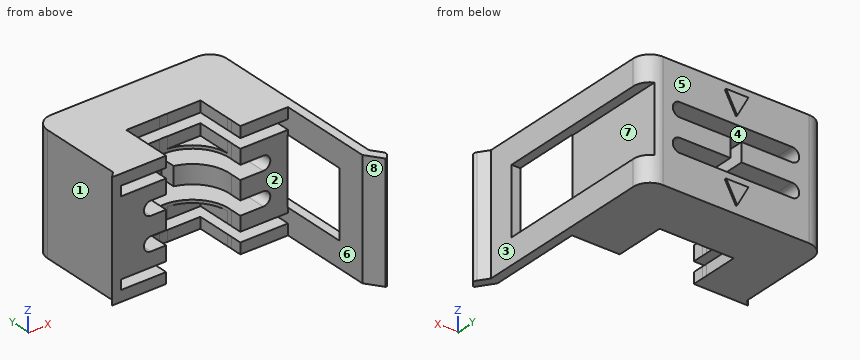
from build123d import *

# Parameters (mm, degrees)
SALIENTE_EXTRUIR1_DEPTH = 21.02
CORTAR_EXTRUIR1_DEPTH   = 48.423848102
SALIENTE_EXTRUIR2_DEPTH = 0.3
CORTAR_EXTRUIR2_DEPTH   = 1.7
CROQUIS6_W              = 13.32
CROQUIS6_H              = 9.1
CORTAR_EXTRUIR3_DEPTH   = 5.78
CROQUIS7_W              = 13.32
CROQUIS7_H              = 9.1
CORTAR_EXTRUIR4_DEPTH   = 5.78
CROQUIS8_W              = 21.89
CROQUIS8_H              = 1.74582909
CORTAR_EXTRUIR5_DEPTH   = 15.76


with BuildPart() as part:
    # Croquis2 → Saliente-Extruir1 (new body)
    with BuildSketch(Plane.XY):
        with BuildLine():
            Line((16.1, -25.6), (16.1, -9.1))
            Line((16.1, -9.1), (16.1, 6.87))
            ThreePointArc((16.1, 6.87), (15.221320344, 8.991320344), (13.1, 9.87))
            Line((13.1, 9.87), (-13.1, 9.87))
            ThreePointArc((-13.1, 9.87), (-15.221320344, 8.991320344), (-16.1, 6.87))
            Line((-16.1, 6.87), (-16.1, -8.084842917))
            Line((-16.1, -8.084842917), (-17.1, -9.1))
            Line((-17.1, -9.1), (-16.1, -9.1))
            Line((-16.1, -9.1), (-7.36, -9.1))
            Line((-7.36, -9.1), (-7.36, -7.1))
            ThreePointArc((-7.36, -7.1), (-0.7, 0.036800452), (5.96, -7.1))
            Line((5.96, -7.1), (5.96, -9.1))
            Line((5.96, -9.1), (14.53, -9.1))
            Line((14.53, -9.1), (14.53, -26.095019099))
            Line((14.53, -26.095019099), (16.46294155, -28.855545721))
            ThreePointArc((16.46294155, -28.855545721), (16.646307517, -28.898064095), (16.810355034, -28.805764032))
            Line((16.810355034, -28.805764032), (16.821593757, -28.791058008))
            Line((16.821593757, -28.791058008), (17.28495009, -28.184749839))
            ThreePointArc((17.28495009, -28.184749839), (17.43599966, -27.735907903), (17.281999232, -27.288069848))
            Line((17.281999232, -27.288069848), (16.1, -25.6))
        make_face()
    extrude(amount=SALIENTE_EXTRUIR1_DEPTH)

    # Croquis3 → Cortar-Extruir1 (cut, through all)
    with BuildSketch(Plane(origin=(0, 9.87, 0), x_dir=(1, 0, 0), z_dir=(0, 1, 0))):
        with BuildLine():
            Line((-10.1, -12.17), (-1, -12.17))
            Line((-1, -12.17), (-1, -8.83))
            Line((-1, -8.83), (-10.1, -8.83))
            ThreePointArc((-10.1, -8.83), (-11.35, -7.58), (-10.1, -6.33))
            Line((-10.1, -6.33), (10.1, -6.33))
            ThreePointArc((10.1, -6.33), (11.35, -7.58), (10.1, -8.83))
            Line((10.1, -8.83), (1, -8.83))
            Line((1, -8.83), (1, -12.17))
            Line((1, -12.17), (10.1, -12.17))
            ThreePointArc((10.1, -12.17), (11.35, -13.42), (10.1, -14.67))
            Line((10.1, -14.67), (-10.1, -14.67))
            ThreePointArc((-10.1, -14.67), (-11.35, -13.42), (-10.1, -12.17))
        make_face()
    extrude(amount=-CORTAR_EXTRUIR1_DEPTH, mode=Mode.SUBTRACT)

    # Croquis4 → Saliente-Extruir2 (add)
    with BuildSketch(Plane(origin=(0, 9.87, 0), x_dir=(-1, 0, 0), z_dir=(0, 1, 0))):
        Polygon((0, 16.02), (2, 19.67), (-2, 19.67), align=None)
        Polygon((2, 4.98), (-2, 4.98), (0, 1.33), align=None)
    extrude(amount=SALIENTE_EXTRUIR2_DEPTH)

    # Croquis5 → Cortar-Extruir2 (cut)
    with BuildSketch(Plane(origin=(16.1, 0, 0), x_dir=(0, 0, -1), z_dir=(1, 0, 0))):
        Polygon((-16.46, 6.87), (-16.46, -20.9), (-10.51, -20.9), (-4.56, -20.9), (-4.56, 6.87), align=None)
        Polygon((-16.46, 9.815378902), (-16.46, 6.87), (-4.56, 6.87), (-4.56, 10.17), align=None)
    extrude(amount=-CORTAR_EXTRUIR2_DEPTH, mode=Mode.SUBTRACT)

    # Croquis6 → Cortar-Extruir3 (cut)
    with BuildSketch(Plane(origin=(0, 0, 0), x_dir=(-1, 0, 0), z_dir=(0, 0, -1))):
        with Locations((0.7, -4.55)):
            Rectangle(CROQUIS6_W, CROQUIS6_H)
    extrude(amount=-CORTAR_EXTRUIR3_DEPTH, mode=Mode.SUBTRACT)

    # Croquis7 → Cortar-Extruir4 (cut)
    with BuildSketch(Plane.XY.offset(21.02)):
        with Locations((-0.7, -4.55)):
            Rectangle(CROQUIS7_W, CROQUIS7_H)
    extrude(amount=-CORTAR_EXTRUIR4_DEPTH, mode=Mode.SUBTRACT)

    # Croquis8 → Cortar-Extruir5 (cut)
    with BuildSketch(Plane.XZ.offset(9.1)):
        Polygon((-7.36, 19.04), (-9.552269286, 19.04), (-15.51, 19.04), (-15.51, 17.29417091), (-9.552269286, 17.29417091), (-7.36, 17.29417091), align=None)
        with Locations((3.585, 18.167085455)):
            Rectangle(CROQUIS8_W, CROQUIS8_H)
        with Locations((3.585, 2.832914545)):
            Rectangle(CROQUIS8_W, CROQUIS8_H)
        Polygon((-15.51, 3.70582909), (-15.51, 1.96), (-9.552269286, 1.96), (-7.36, 1.96), (-7.36, 3.70582909), (-9.552269286, 3.70582909), align=None)
    extrude(amount=-CORTAR_EXTRUIR5_DEPTH, mode=Mode.SUBTRACT)


solid = part.part
Geometry check sheet. Reference: the model listing, model coordinates, mm. Face numbers are marked on the shaded views. A direction names the side the tool comes from. Coordinates: 2 decimals unless noted, no trailing zeros. Write each loop counter-clockwise with the first axis right and the second up, starting at its lowest first coordinate (ties: lowest second). Pieces come first, ordered by that corner, then holes. Notation, with made-up numbers: (73, 29) -> (118, 29) arc R27 cw to (118, 50) -> close; hole circle Ø3 at (53, -21). An arc over 180 degrees is marked (long way). One line per question, with ' | ' between items.
1. Set-up check for the marked faces 1, 2, 3 and 4: record each of +Z, -Z, +X, -X, +Y, -Y from which the full face is reachable in a straight line by a thin tool's end or side.
Answers:
face 1: +Z, -Z, -X, +Y | face 2: +Z, -Z, -X, -Y | face 3: +Z, -Z, +X, +Y | face 4: +Y, -Y
2. Cross-section at B-B on y = 4.5. Record the cut outline in (x, z).
Answers:
outline: (-16.1, 0) -> (16.1, 0) -> (16.1, 4.56) -> (14.4, 4.56) -> (14.4, 16.46) -> (16.1, 16.46) -> (16.1, 21.02) -> (-16.1, 21.02) -> close; hole (-15.51, 1.96) -> (14.53, 1.96) -> (14.53, 3.71) -> (-15.51, 3.71) -> close; hole (-15.51, 17.29) -> (14.53, 17.29) -> (14.53, 19.04) -> (-15.51, 19.04) -> close; hole (-10.1, 6.33) -> (10.1, 6.33) arc R1.25 ccw to (10.1, 8.83) -> (1, 8.83) -> (1, 12.17) -> (10.1, 12.17) arc R1.25 ccw to (10.1, 14.67) -> (-10.1, 14.67) arc R1.25 ccw to (-10.1, 12.17) -> (-1, 12.17) -> (-1, 8.83) -> (-10.1, 8.83) arc R1.25 ccw to start
3. Cross-section at A-A on z = 7.58. Record the cut outline in (x, y).
Answers:
outline: (-17.1, -9.1) -> (-11.35, -9.1) -> (-11.35, 9.87) -> (-13.1, 9.87) arc R3 ccw to (-16.1, 6.87) -> (-16.1, -8.08) -> close; (11.35, -9.1) -> (14.4, -9.1) -> (14.4, 9.57) arc R3 ccw to (13.1, 9.87) -> (11.35, 9.87) -> close; (14.53, -26.1) -> (16.46, -28.86) arc R0.26 ccw to (16.81, -28.81) -> (17.28, -28.18) arc R0.74 ccw to (17.28, -27.29) -> (16.1, -25.6) -> (16.1, -20.9) -> (14.53, -20.9) -> close
4. Cross-section at D-D on x = 5.5. Record the cut outline in (y, z).
Answers:
outline: (-4.16, 5.78) -> (0, 5.78) -> (0, 3.71) -> (6.66, 3.71) -> (6.66, 1.96) -> (0, 1.96) -> (0, 0) -> (9.87, 0) -> (9.87, 6.33) -> (-4.16, 6.33) -> close; (-4.16, 8.83) -> (9.87, 8.83) -> (9.87, 12.17) -> (-4.16, 12.17) -> close; (-4.16, 14.67) -> (9.87, 14.67) -> (9.87, 21.02) -> (0, 21.02) -> (0, 19.04) -> (6.66, 19.04) -> (6.66, 17.29) -> (0, 17.29) -> (0, 15.24) -> (-4.16, 15.24) -> close
5. Thickness scan on probe 1 along Z at (x, y) = (9, -2.5); probe 2 along Z at (x, y) = (11.5, 6.5); probe 3 along X at (y, z) = (-7.5, 15). Record the ranges inside material, lowest first. Write a range as from..to.
Answers:
probe 1: z = 0..1.96, 3.71..6.33, 8.83..12.17, 14.67..17.29, 19.04..21.02 | probe 2: z = 0..1.96, 3.71..17.29, 19.04..21.02 | probe 3: x = -16.1..-7.36, 5.96..14.4
6. Cross-section at C-C on x = -9.5. Record the cut outline in (y, z).
Answers:
outline: (-9.1, 0) -> (9.87, 0) -> (9.87, 6.33) -> (-9.1, 6.33) -> (-9.1, 3.71) -> (6.66, 3.71) -> (6.66, 1.96) -> (-9.1, 1.96) -> close; (-9.1, 8.83) -> (9.87, 8.83) -> (9.87, 12.17) -> (-9.1, 12.17) -> close; (-9.1, 14.67) -> (9.87, 14.67) -> (9.87, 21.02) -> (-9.1, 21.02) -> (-9.1, 19.04) -> (6.66, 19.04) -> (6.66, 17.29) -> (-9.1, 17.29) -> close
7. Depth check by flat-ended pin: pin 1 Ø4 at (x, z) = (7, 13) entering from -Y; pin 2 Ø9.5 at (x, y) = (-1.5, 4) entering from -Z; pin 3 Ø1 at (y, z) = (-7.5, 20.5) entering from +X; pin 4 Ø1 at (y, z) = (-3, 5) entering from -X. Enter the tip coordinate at first touch or a pass-through.
Answers:
pin 1: stops at y = -9.1 | pin 2: stops at z = 0 | pin 3: stops at x = 16.1 | pin 4: stops at x = -16.1
8. Draft check along X on the marked faces 5, 6, 7 and 8. Enter one of: +X half, -X half, draft (parallel to the pull), parting line (faces both ways), or undercut.
Answers:
face 5: draft | face 6: undercut | face 7: +X half | face 8: -X half
